from build123d import *

# Parameters (mm, degrees)
F0_W          = 7.9684891073
F0_H          = 62.2722776352
F1_DEPTH      = 6.35
F2_R          = 7.62
F3_R          = 12.7
F4_W          = 5.0514815375
F4_H          = 28.3501516096
F5_DEPTH      = 7.62
F5_DEPTH_BACK = 1.27
F6_R          = 0.508
F7_R          = 0.508
F8_R          = 0.508
F9_R          = 5.08


with BuildPart() as f1:
    # F0 (on Front) → F1 (new body)
    with BuildSketch(Plane.XZ):
        with Locations((-13.4939518757, 12.9458873377)):
            Rectangle(F0_W, F0_H)
        with BuildLine():
            ThreePointArc((-23.2001595007, 59.7813798143), (-22.7239205368, 51.0625328759), (-17.4781964294, 44.0820261553))
            Line((-17.4781964294, 44.0820261553), (-9.5097073221, 44.0820261553))
            ThreePointArc((-9.5097073221, 44.0820261553), (-4.2639832147, 51.0625328759), (-3.7877442507, 59.7813798143))
            Line((-3.7877442507, 59.7813798143), (-7.1439518757, 59.7813798143))
            Line((-7.1439518757, 59.7813798143), (-7.1439518757, 50.6561658404))
            Line((-7.1439518757, 50.6561658404), (-9.5097073221, 47.7606636927))
            Line((-9.5097073221, 47.7606636927), (-17.4781964294, 47.7606636927))
            Line((-17.4781964294, 47.7606636927), (-19.8439518757, 50.6561658404))
            Line((-19.8439518757, 50.6561658404), (-19.8439518757, 59.7813798143))
            Line((-19.8439518757, 59.7813798143), (-23.2001595007, 59.7813798143))
        make_face()
        Polygon((-19.8439518757, 64.6756440401), (-23.2001595007, 59.7813798143), (-19.8439518757, 59.7813798143), align=None)
        Polygon((-7.1439518757, 59.7813798143), (-3.7877442507, 59.7813798143), (-7.1439518757, 64.6756440401), align=None)
    extrude(amount=F1_DEPTH)

    # F2
    f2_edges = [f1.edges().sort_by_distance(p)[0] for p in [
        (-17.478196, -3.175, 44.082026),
    ]]
    fillet(f2_edges, radius=F2_R)

    # F3
    f3_edges = [f1.edges().sort_by_distance(p)[0] for p in [
        (-3.787744, -3.175, 59.78138),
        (-23.20016, -3.175, 59.78138),
    ]]
    fillet(f3_edges, radius=F3_R)

    # F4 (on face) → F5 (join, two sides)
    with BuildSketch(Plane(origin=(0, 0, 0), x_dir=(-1, 0, 0), z_dir=(0, 1, 0))) as f5_sk:
        with Locations((13.6485905387, 12.7843844239)):
            Rectangle(F4_W, F4_H)
    extrude(amount=-F5_DEPTH)
    extrude(f5_sk.sketch, amount=F5_DEPTH_BACK)

    # F6
    f6_edges = [f1.edges().sort_by_distance(p)[0] for p in [
        (-11.12285, 0, 12.784384),
        (-13.648591, 0, -1.390691),
        (-13.648591, 0, 26.95946),
        (-16.174331, 0, 12.784384),
    ]]
    fillet(f6_edges, radius=F6_R)

    # F7
    f7_edges = [f1.edges().sort_by_distance(p)[0] for p in [
        (-11.12285, 1.27, 12.784384),
        (-13.648591, 1.27, -1.390691),
        (-16.174331, 1.27, 12.784384),
        (-13.648591, 1.27, 26.95946),
    ]]
    fillet(f7_edges, radius=F7_R)

    # F8
    f8_edges = [f1.edges().sort_by_distance(p)[0] for p in [
        (-13.648591, -6.35, -1.390691),
        (-11.12285, -6.35, 12.784384),
        (-13.648591, -6.35, 26.95946),
        (-16.174331, -6.35, 12.784384),
        (-11.12285, -7.62, 12.784384),
        (-13.648591, -7.62, -1.390691),
        (-16.174331, -7.62, 12.784384),
        (-13.648591, -7.62, 26.95946),
    ]]
    fillet(f8_edges, radius=F8_R)

    # F9
    f9_edges = [f1.edges().sort_by_distance(p)[0] for p in [
        (-9.509707, -3.175, 44.082026),
    ]]
    fillet(f9_edges, radius=F9_R)


solid = f1.part
Verification items for the finished model (mm, model axes). A direction names the side the tool comes from. Give positions to 0.01 mm unless a question says otherwise; leave off trailing zeros. Write each loop counter-clockwise with the first axis right and the second up, starting at its lowest first coordinate (ties: lowest second). Pieces come first, ordered by that corner, then holes. Notation, with made-up numbers: M -11,38.5 L 46,38.5 A22 cw 46,60.5 Z; hole C -10.5,80 d1. An arc over 180 degrees is marked long. Put each result on its own line as item: value. Start each with the question number.
1. Section check B-B (z = 56). Record the cut outline in (x, y).
2. Go/stop test with flat-tipped pins: pin 1 Ø1 at (x, y) = (-16.5, -5) entering from +Z; pin 2 Ø2 at (x, y) = (-21, -0.5) entering from +Z; pin 3 Ø1.9 at (y, z) = (-3.5, 3.5) entering from -X. Record where each tip stops, or that it passes through.
3. Section check A-A (y = -1.5). Record the cut outline in (x, z), and give its area (3 significant figures).
4. Draft check along X on faces 1 (the face through (-18.645, -3.131, 49.188)), 2 (the face through (-19.844, -3, 58)), 3 (the face through (-14, -3, -18.19)), 4 (the face through (-18, -3.22, 43.46)). Enter one of: +X half, -X half, draft (parallel to the pull), parting line (faces both ways), or undercut.
5. Scan lines: line 1 along X through (y, z) = (-3, 10.5); line 2 along Z through (x, y) = (-11.25, -3); line 3 along Y through (x, z) = (-15.5, -3.5). Record each from-to range of solid material in increasing order. Write a range as [from, to].
6. Set-up check for faces 5 (the face through (-7.144, -3, 58)), 6 (the face through (-9.51, -3, 11)), 7 (the face through (-17.478, -3, 11)): record each of +Z, -Z, +X, -X, +Y, -Y from which the full face is reachable in a straight line by a thin tool's end or side.
7. Section check D-D (z = 25). Record the cut outline in (x, y).
8. Section check C-C (x = -13.25). Record the cut outline in (y, z).
Answer list:
1. outline: M -23.48,-6.35 L -19.84,-6.35 L -19.84,0 L -23.48,0 Z; M -7.14,-6.35 L -3.51,-6.35 L -3.51,0 L -7.14,0 Z
2. pin 1: z = 47.76
2. pin 2: z = 64.45
2. pin 3: x = -17.48
3. outline: M -22.74,51.1 A15.02 ccw -19.55,45.91 A7.62 cw -17.48,40.69 L -17.48,-18.19 L -9.51,-18.19 L -9.51,41.73 A5.08 cw -7.95,45.39 A15.02 ccw -4.25,51.1 A12.7 ccw -5.72,62.6 L -7.14,64.68 L -7.14,50.66 L -9.51,47.76 L -17.48,47.76 L -19.84,50.66 L -19.84,64.68 L -21.27,62.6 A12.7 ccw Z
3. area: 638 mm2
4. face 1: undercut
4. face 2: undercut
4. face 3: draft
4. face 4: -X half
5. line 1: [-17.48, -9.51]
5. line 2: [-18.19, 47.76]
5. line 3: [-6.35, 0]
6. face 5: +Z, +Y, -Y
6. face 6: -Z, +X, +Y, -Y
6. face 7: -Z, -X, +Y, -Y
7. outline: M -17.48,-6.35 L -16.68,-6.35 A0.51 cw -16.17,-6.86 L -16.17,-7.11 A0.51 ccw -15.67,-7.62 L -11.63,-7.62 A0.51 ccw -11.12,-7.11 L -11.12,-6.86 A0.51 cw -10.61,-6.35 L -9.51,-6.35 L -9.51,0 L -10.61,0 A0.51 cw -11.12,0.51 L -11.12,0.76 A0.51 ccw -11.63,1.27 L -15.67,1.27 A0.51 ccw -16.17,0.76 L -16.17,0.51 A0.51 cw -16.68,0 L -17.48,0 Z
8. outline: M -7.62,-0.88 A0.51 ccw -7.11,-1.39 L -6.86,-1.39 A0.51 cw -6.35,-1.9 L -6.35,-18.19 L 0,-18.19 L 0,-1.9 A0.51 cw 0.51,-1.39 L 0.76,-1.39 A0.51 ccw 1.27,-0.88 L 1.27,26.45 A0.51 ccw 0.76,26.96 L 0.51,26.96 A0.51 cw 0,27.47 L 0,47.76 L -6.35,47.76 L -6.35,27.47 A0.51 cw -6.86,26.96 L -7.11,26.96 A0.51 ccw -7.62,26.45 Z
